For this review, use the dimensioned drawing (mm, ordinates from the lowest corner) and the shaded views. A direction names the side the tool comes from. Give positions to 0.01 mm unless a question says otherwise; leave off trailing zeros. Order: outer loops, then holes, each group sorted by start corner. A loop starts at its lowest first (then second) coordinate and runs counter-clockwise, first axis right, second up. Notation, with made-up numbers: (30, -24) - (50, -24) arc R35 ccw to (50, 8) - close; hole circle Ø6 at (-30.75, -28). An arc over 180 degrees is marked (long way). Use a Markdown table: item, result. Add a question column.
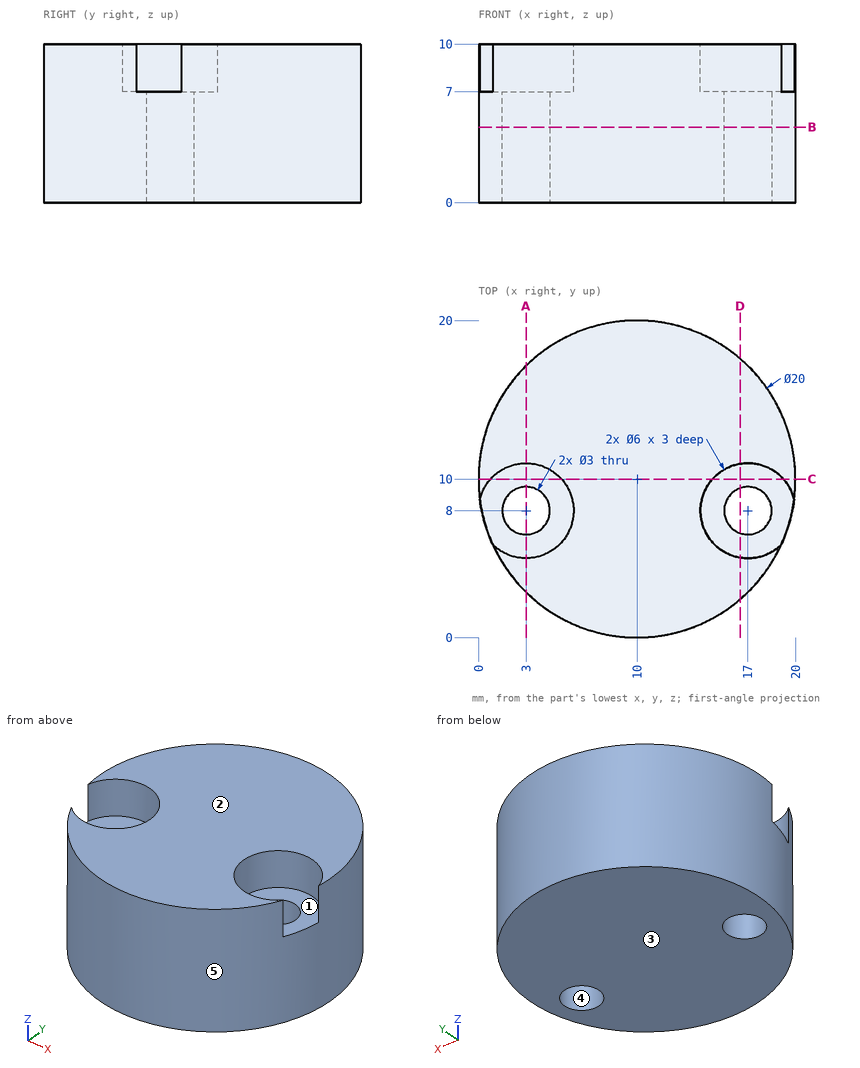
Q1. We need section B-B (z = 4.75). Write out the cut boundary in (x, y), plus the area to 3 significant figures.
Q2. Machinability: for the marked faces 1 and 2, which of the approach directions +Z, -Z, +X, -X, +Y, -Y give a long, thin tool a straight path to every point of the face, cutting with its end or side? Answer none if there is none.
Q3. We need section A-A (x = 3). Write out the cut boundary in (y, z), plus the area to 3 significant figures.
Q4. Draft analysis for pull direction X (two halves, no side actions). For the marked faces 3, 4 and 5, state which applies: pulls with the +X half, pulls with the -X half, needs draft (parallel to the pull), parting line crosses it, or undercut.
Q5. We need section C-C (y = 10). Write out the cut boundary in (x, z).
Q6. We need section D-D (x = 16.5). Write out the cut boundary in (y, z).
Q7. Wall thickness on probe 1 along X at (y, z) = (8.5, 2.75); probe 2 along X at (y, z) = (7.5, 2.5); probe 3 along X at (y, z) = (8, 7.6): over which ranges is each line inside the solid? List them lowest first.
Q8. Clearance check with flat-ended pins moving along their axes: P1, Ø1.5, axis at x = 17.5, z = 6, coming from the -Y side; P2, Ø6, axis at y = 4, z = 4.5, coming from the +X side; P3, Ø2, axis at x = 14.5, z = 2, coming from the -Y side. State where each tip first meets the part, or that it passes through.
Here are the results:
| question | item | result |
|---|---|---|
| 1 | outline | circle Ø20 at (10, 10); hole circle Ø3 at (3, 8); hole circle Ø3 at (17, 8) |
| 1 | area | 300 mm2 |
| 2 | face 1 | +Z |
| 2 | face 2 | +Z, +X, -X, +Y, -Y |
| 3 | outline | (2.86, 0) - (6.5, 0) - (6.5, 7) - (5, 7) - (5, 10) - (2.86, 10) - close; (9.5, 0) - (17.14, 0) - (17.14, 10) - (11, 10) - (11, 7) - (9.5, 7) - close |
| 3 | area | 104 mm2 |
| 4 | face 3 | needs draft |
| 4 | face 4 | undercut |
| 4 | face 5 | parting line crosses it |
| 5 | outline | (0, 0) - (20, 0) - (20, 10) - (19.24, 10) - (19.24, 7) - (14.76, 7) - (14.76, 10) - (5.24, 10) - (5.24, 7) - (0.76, 7) - (0.76, 10) - (0, 10) - close |
| 6 | outline | (2.4, 0) - (6.59, 0) - (6.59, 7) - (5.04, 7) - (5.04, 10) - (2.4, 10) - close; (9.41, 0) - (17.6, 0) - (17.6, 10) - (10.96, 10) - (10.96, 7) - (9.41, 7) - close |
| 7 | probe 1 | 0.11 to 1.59, 4.41 to 15.59, 18.41 to 19.89 |
| 7 | probe 2 | 0.32 to 1.59, 4.41 to 15.59, 18.41 to 19.68 |
| 7 | probe 3 | 6 to 14 |
| 8 | P1 | y = 2.62 |
| 8 | P2 | x = 19.54 |
| 8 | P3 | y = 0.63 |
